Could you check a few things on this model? Use its own coordinates, in mm. A direction names the side the tool comes from. Round coordinates to 2 decimals unless told otherwise and drop trailing zeros. Loops run counter-clockwise (first coordinate to the right, second up) from the corner with the lowest first, then second, coordinate; pieces in that order, holes last. Notation, with made-up numbers: M 25,-1.5 L 40,-1.5 A19 cw 40,26.5 Z; hole C -13,-3.5 d9. An arc over 180 degrees is marked long. One line per item, written item: value. Start each with the question number.
Q1. Please list where these lines run through material, in increasing order: line 1 along X through (y, z) = (5, 0); line 2 along Y through (x, z) = (-9.75, 1.25); line 3 along X through (y, z) = (-0.5, -7.25).
Q2. Thinking about a two-plate mould opening in X: for faces 1 (the face through (-10.74, 9.91, -2.38)), 2 (the face through (0, 0, -10)), 3 (the face through (-7.81, 4.41, 1.73)), which applies, released by +X, released by -X, zero draft, split by the parting line, or undercut?
Q3. I'm going to push flat-ended pins straight in: pin 1 Ø4 at (x, y) = (-1, 5) entering from +Z; pin 2 Ø1 at (x, y) = (-4.5, 1) entering from -Z; pin 3 Ø1.5 at (x, y) = (8, 4) entering from +Z; pin 4 Ø13 at (x, z) = (0, 0) entering from -Y (3 decimals). Where does each tip first touch, or does it pass through?
Q4. Imagine slicing it at A-A (x = 0). Please give me the cut outline in (y, z).
Q5. Imagine slicing it at B-B (z = 0). Please give me the cut outline in (x, y).
Q6. Imagine slicing it at C-C (y = -1). Please give me the cut outline in (x, z), then the cut area to 3 significant figures.
Q7. Which directions (+Z, -Z, +X, -X, +Y, -Y) give clear straight access to the entire face, cutting with the end or side of a thin tool? Please do faces 4 (the face through (10.74, -0.94, -2.38)), 5 (the face through (0, 9, -10)).
from build123d import *

# Parameters (mm, degrees)
SKETCH1_R           = 8.5
BOSS_EXTRUDE1_DEPTH = 9
SKETCH2_R           = 11
BOSS_EXTRUDE2_DEPTH = 1.85
BOSS_EXTRUDE4_START = 1.85
SKETCH4_R           = 11
BOSS_EXTRUDE4_DEPTH = 1.85
SKETCH5_R           = 8
CUT_EXTRUDE1_DEPTH  = 21.082081565
FILLET1_R           = 1


with BuildPart() as part:
    # Sketch1 → Boss-Extrude1 (new body)
    with BuildSketch(Plane(origin=(0, 0, 0), x_dir=(1, 0, 0), z_dir=(0, 1, 0))):
        with Locations(Location((0, 0, 0), (0, 0, 270))):
            Circle(SKETCH1_R)
    extrude(amount=BOSS_EXTRUDE1_DEPTH)

    # Sketch2 → Boss-Extrude2 (add)
    with BuildSketch(Plane(origin=(0, 9, 0), x_dir=(1, 0, 0), z_dir=(0, 1, 0))):
        with Locations(Location((0, 0, 0), (0, 0, 270))):
            Circle(SKETCH2_R)
    extrude(amount=BOSS_EXTRUDE2_DEPTH)

    # Sketch4 → Boss-Extrude4 (add)
    with BuildSketch(Plane.XZ.offset(BOSS_EXTRUDE4_START)):
        with Locations(Location((0, 0, 0), (0, 0, 90))):
            Circle(SKETCH4_R)
    extrude(amount=-BOSS_EXTRUDE4_DEPTH)

    # Sketch5 → Cut-Extrude1 (cut, through all)
    with BuildSketch(Plane.XZ.offset(1.85)):
        with Locations(Location((0, 0, 0), (0, 0, 270))):
            Circle(SKETCH5_R)
    extrude(amount=-CUT_EXTRUDE1_DEPTH, mode=Mode.SUBTRACT)

    # Fillet1
    fillet1_edges = [part.edges().sort_by_distance(p)[0] for p in [
        (0, 0, -8.5),
        (0, 9, -8.5),
    ]]
    fillet(fillet1_edges, radius=FILLET1_R)


solid = part.part
Report:
1. line 1: x = -8.5 to -8, 8 to 8.5
1. line 2: y = -1.85 to 0, 9 to 10.85
1. line 3: x = -8.27 to -3.38, 3.38 to 8.27
2. face 1: split by the parting line
2. face 2: zero draft
2. face 3: undercut
3. pin 1: stops at z = 8.5
3. pin 2: stops at z = -7.5
3. pin 3: stops at z = 4.44
3. pin 4: passes through
4. outline: M -1.85,-11 L 0,-11 L 0,-9.5 A1 cw 1,-8.5 L 8,-8.5 A1 cw 9,-9.5 L 9,-11 L 10.85,-11 L 10.85,-8 L -1.85,-8 Z; M -1.85,8 L 10.85,8 L 10.85,11 L 9,11 L 9,9.5 A1 cw 8,8.5 L 1,8.5 A1 cw 0,9.5 L 0,11 L -1.85,11 Z
5. outline: M -11,-1.85 L -8,-1.85 L -8,10.85 L -11,10.85 L -11,9 L -9.5,9 A1 cw -8.5,8 L -8.5,1 A1 cw -9.5,0 L -11,0 Z; M 8,-1.85 L 11,-1.85 L 11,0 L 9.5,0 A1 cw 8.5,1 L 8.5,8 A1 cw 9.5,9 L 11,9 L 11,10.85 L 8,10.85 Z
6. outline: C 0,0 d22; hole C 0,0 d16
6. area: 179 mm²
7. face 4: +Y, -Y
7. face 5: none
